Can you work these out from the model? Positions are in its coordinate system, mm. Round coordinates to 2 decimals unless told otherwise and drop trailing zeros. Loops run counter-clockwise (first coordinate to the right, second up) from the corner with the lowest first, then second, coordinate; pieces in that order, holes last.
```python
from build123d import *

# Parameters (mm, degrees)
BOSS_EXTRUDE1_DEPTH = 40
SKETCH2_R           = 1.5
CUT_EXTRUDE1_DEPTH  = 40
SKETCH3_R           = 1.5
CUT_EXTRUDE2_DEPTH  = 40


with BuildPart() as part:
    # Sketch1 → Boss-Extrude1 (new body)
    with BuildSketch(Plane.XY):
        with BuildLine():
            Line((0, 0), (-9.98617259, 21.415416229))
            ThreePointArc((-9.98617259, 21.415416229), (-13.676254377, 25.623148069), (-19.04925046, 27.189233611))
            Line((-19.04925046, 27.189233611), (-52.678547852, 27.189233611))
            Line((-52.678547852, 27.189233611), (-52.678547852, 33.189233611))
            Line((-52.678547852, 33.189233611), (-19.04925046, 33.189233611))
            ThreePointArc((-19.04925046, 33.189233611), (-10.452456727, 30.683496744), (-4.548325868, 23.951125799))
            Line((-4.548325868, 23.951125799), (5.437846722, 2.53570957))
            Line((5.437846722, 2.53570957), (0, 0))
        make_face()
    extrude(amount=BOSS_EXTRUDE1_DEPTH)

    # Sketch2 → Cut-Extrude1 (cut)
    with BuildSketch(Plane(origin=(0, 33.189233611, 0), x_dir=(1, 0, 0), z_dir=(0, 1, 0))):
        with Locations(Location((-35.863899156, -15, 0), (0, 0, 270))):
            Circle(SKETCH2_R)
        with Locations(Location((-35.863899156, -25, 0), (0, 0, 270))):
            Circle(SKETCH2_R)
    extrude(amount=-CUT_EXTRUDE1_DEPTH, mode=Mode.SUBTRACT)

    # Sketch3 → Cut-Extrude2 (cut)
    with BuildSketch(Plane(origin=(5.437846722, 2.53570957, 0), x_dir=(0, 0, -1), z_dir=(0.906307787036651, 0.42261826174069705, 0))):
        with Locations(Location((-15, 11.814648696, 0), (0, 0, 90))):
            Circle(SKETCH3_R)
        with Locations(Location((-25, 11.814648696, 0), (0, 0, 90))):
            Circle(SKETCH3_R)
    extrude(amount=-CUT_EXTRUDE2_DEPTH, mode=Mode.SUBTRACT)


solid = part.part
```
(1) Suppose I cut it at D-D (y = 8.5). Write out the boundary of the cut face in (x, z).
(2) If I drill on line 1 (Y direction, x = -19, z = 20); line 2 (X direction, y = 30, z = 24.5); line 3 (X direction, y = 31.15, z = 25), over which ranges is the centre line in solid material (lowest first)?
(3) Suppose I cut it at A-A (z = 15). Write out the boundary of the cut face in (x, y), then the cut area to 3 significant figures.
(4) Suppose I cut it at C-C (x = -43.5). Write out the boundary of the cut face in (y, z).
(5) Suppose I cut it at B-B (z = 36.5). Write out the boundary of the cut face in (x, y), then the cut area to 3 significant figures.
(6) We'd pull the mould along Y, two halves only. Please class faces 1 (the cylindrical face through (-36.78, 30.23, 13.81)), 2 (the cylindrical face through (-2.154, 11.816, 26.487)), 3 (the flat face through (-36, 27.189, 20)): released by +Y, released by -Y, zero draft, split by the parting line, or undercut.
(7) For pin 1 (2 mm diameter, centred on x = -7, z = 35.5, fed in from -Y); pin 2 (2.5 mm diameter, centred on x = -35.86, z = 15, fed in from -Y); pin 3 (10 mm diameter, centred on x = -38.5, z = 24.5, fed in from -Y); pin 4 (10 mm diameter, centred on x = -1.5, z = 4, fed in from -Y), each with a flat end and sliding along its axis, tell me the tip position at first contact or that it passes through.
Check result:
1. outline: (-3.96, 0) - (2.66, 0) - (2.66, 40) - (-3.96, 40) - close
2. line 1: y = 27.19 to 33.19
2. line 2: x = -52.68 to -37.28, -34.45 to -9.46
2. line 3: x = -52.68 to -37.36, -34.36 to -11.23
3. outline: (-52.68, 27.19) - (-37.36, 27.19) - (-37.36, 33.19) - (-52.68, 33.19) - close; (-34.36, 27.19) - (-19.05, 27.19) arc R10 cw to (-9.99, 21.42) - (-5.63, 12.07) - (-0.19, 14.6) - (-4.55, 23.95) arc R16 ccw to (-19.05, 33.19) - (-34.36, 33.19) - close; (-4.36, 9.35) - (0, 0) - (5.44, 2.54) - (1.08, 11.88) - close
3. area: 396 mm2
4. outline: (27.19, 0) - (33.19, 0) - (33.19, 40) - (27.19, 40) - close
5. outline: (-52.68, 27.19) - (-19.05, 27.19) arc R10 cw to (-9.99, 21.42) - (0, 0) - (5.44, 2.54) - (-4.55, 23.95) arc R16 ccw to (-19.05, 33.19) - (-52.68, 33.19) - close
5. area: 432 mm2
6. face 1: zero draft
6. face 2: undercut
6. face 3: released by -Y
7. pin 1: stops at y = 12.87
7. pin 2: passes through
7. pin 3: stops at y = 27.19
7. pin 4: stops at y = 0
